from build123d import *

# Parameters (mm, degrees)
ESQUISSE1_R      = 40
ESQUISSE1_R_2    = 34
EXTRUSION1_DEPTH = 50
EXTRUSION2_DEPTH = 5


with BuildPart() as part:
    # Esquisse1 → Extrusion1 (new body)
    with BuildSketch(Plane(origin=(0, 0, 0), x_dir=(1, 0, 0), z_dir=(0, 1, 0))):
        Circle(ESQUISSE1_R)
        Circle(ESQUISSE1_R_2, mode=Mode.SUBTRACT)
    extrude(amount=EXTRUSION1_DEPTH)

    # Esquisse2 → Extrusion2 (cut)
    with BuildSketch(Plane(origin=(0, 50, 0), x_dir=(1, 0, 0), z_dir=(0, 1, 0))):
        with BuildLine():
            Line((0, -40), (0, -34))
            ThreePointArc((0, -34), (-1.000433182, -33.985278187), (-2, -33.941125497))
            Line((-2, -33.941125497), (-2.352941176, -39.930735879))
            ThreePointArc((-2.352941176, -39.930735879), (-1.176980214, -39.98268022), (0, -40))
        make_face()
        with BuildLine():
            Line((0, 40), (0, 34))
            ThreePointArc((0, 34), (1.000433182, 33.985278187), (2, 33.941125497))
            Line((2, 33.941125497), (2.352941176, 39.930735879))
            ThreePointArc((2.352941176, 39.930735879), (1.176980214, 39.98268022), (0, 40))
        make_face()
        with BuildLine():
            Line((24.395604074, 31.699440088), (20.736263463, 26.944524075))
            ThreePointArc((20.736263463, 26.944524075), (21.519778552, 26.322977245), (22.284673889, 25.678654748))
            Line((22.284673889, 25.678654748), (26.217263399, 30.210182057))
            ThreePointArc((26.217263399, 30.210182057), (25.317386532, 30.968208524), (24.395604074, 31.699440088))
        make_face()
        with BuildLine():
            Line((-22.489530894, -33.079011475), (-19.11610126, -28.117159754))
            ThreePointArc((-19.11610126, -28.117159754), (-19.934806548, -27.542757449), (-20.736263463, -26.944524075))
            Line((-20.736263463, -26.944524075), (-24.395604074, -31.699440088))
            ThreePointArc((-24.395604074, -31.699440088), (-23.452713586, -32.403244058), (-22.489530894, -33.079011475))
        make_face()
    extrude(amount=-EXTRUSION2_DEPTH, mode=Mode.SUBTRACT)


solid = part.part
Part model, mm, in its own coordinate system. A direction names the side the tool comes from. Coordinates: 2 decimals unless noted, no trailing zeros. Loops run counter-clockwise (first coordinate to the right, second up) from the corner with the lowest first, then second, coordinate; pieces in that order, holes last. Notation, with made-up numbers: (4.25, 48) -> (9.25, 48) arc R23 cw to (9.25, 83) -> close; hole circle Ø6 at (-12, 28.25). An arc over 180 degrees is marked (long way). Use a Markdown table: item, result. Add a question column.
Item 1: Flat gauge pins, fed straight in: P1, Ø4, axis at y = 47, z = -37, coming from the +X side; P2, Ø10, axis at y = 17, z = 9.5, coming from the -X side; P3, Ø12, axis at y = 6.5, z = -30.5, coming from the -X side; P4, Ø10, axis at x = -27.5, z = -2, coming from the +Y side. Where does each tip first touch, or does it go through?
Item 2: Which spindle directions (+Z, -Z, +X, -X, +Y, -Y) get a long thin tool onto all of the face, cutting with end or side? Do faces 5 (the flat face through (0, 48, 37)), 6 (the flat face through (0, 48, -37)), 7 (the flat face through (-20.826, 47.535, 30.633)). Say none if no direction does.
Item 3: Band-saw the part on C-C on y = 22. Write the cut outline in (x, z).
Item 4: Pull direction Z, two halves, no side cores. Call faces 1 (the flat face through (32, 50, 13)), 2 (the cylindrical face through (18.28, 24.65, -28.67)), 3 (the flat face through (22.592, 47.535, -29.355)), 4 (the flat face through (-2.174, 47.535, 36.894)): +Z half, -Z half, draft (parallel to the pull), parting line (faces both ways), or undercut.
Item 5: Band-saw the part on B-B on x = 30. Write the cut outline in (y, z), plus the area to 3 significant figures.
Item 6: Band-saw the part on A-A on z = 0. Write the cut outline in (x, y).
Item 7: Probe probe 1 along X at (y, z) = (37.5, 0); probe 2 along X at (y, z) = (17.5, 3). List the from-to ranges inside material, lowest first.
Geometry says:
| question | item | result |
|---|---|---|
| 1 | P1 | x = 19.36 |
| 1 | P2 | x = -39.75 |
| 1 | P3 | x = -31.62 |
| 1 | P4 | through |
| 2 | face 5 | +Z, +Y |
| 2 | face 6 | -Z, +Y |
| 2 | face 7 | +Y |
| 3 | outline | circle Ø80 at (0, 0); hole circle Ø68 at (0, 0) |
| 4 | face 1 | draft |
| 4 | face 2 | undercut |
| 4 | face 3 | undercut |
| 4 | face 4 | +Z half |
| 5 | outline | (0, -26.46) -> (50, -26.46) -> (50, -16) -> (0, -16) -> close; (0, 16) -> (50, 16) -> (50, 26.46) -> (0, 26.46) -> close |
| 5 | area | 1,050 mm² |
| 6 | outline | (-40, 0) -> (-34, 0) -> (-34, 50) -> (-40, 50) -> close; (34, 0) -> (40, 0) -> (40, 50) -> (34, 50) -> close |
| 7 | probe 1 | -40 to -34, 34 to 40 |
| 7 | probe 2 | -39.89 to -33.87, 33.87 to 39.89 |
